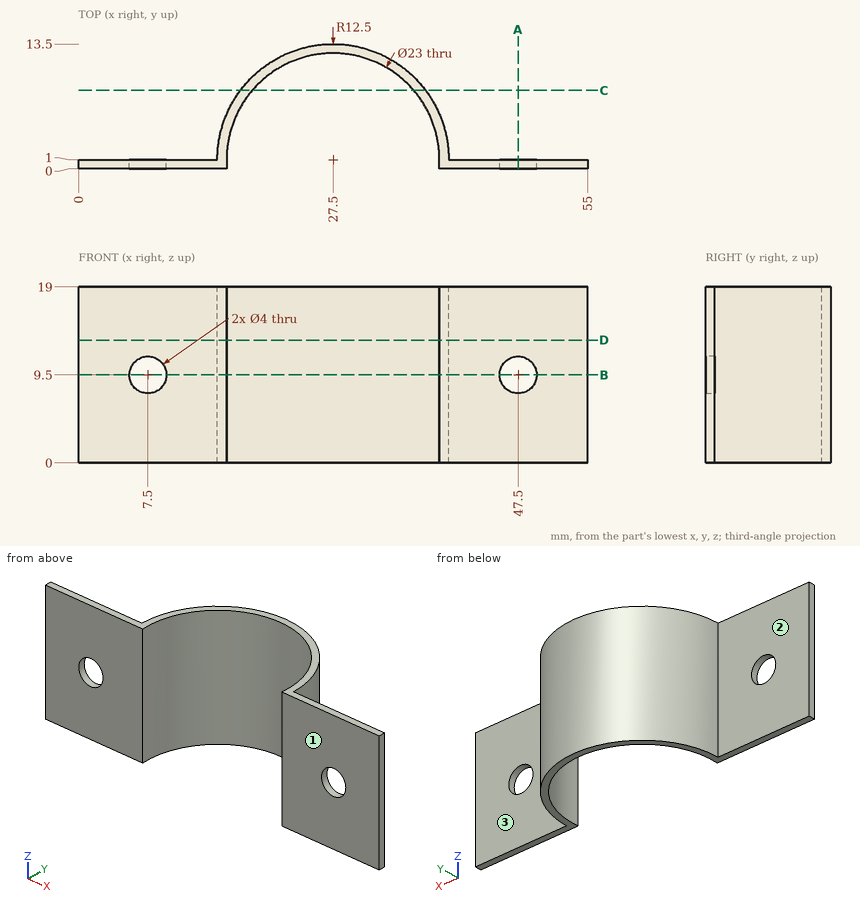
Job drawing, mm, ordinate dimensions from the low corner. One solid piece. A direction names the side the tool comes from. Give positions to 0.01 mm unless a question says otherwise; leave off trailing zeros. Write each loop counter-clockwise with the first axis right and the second up, starting at its lowest first coordinate (ties: lowest second). Pieces come first, ordered by that corner, then holes. Notation, with made-up numbers: M -21,-38.75 L 8,-38.75 A30 ccw 8,-4.75 Z; hole C 65,38.25 d7. An arc over 180 degrees is marked long. Put each result on its own line as item: value. Start each with the question number.
(1) Band-saw the part on B-B, the plane z = 9.5. Write the cut outline in (x, y), and give its area (3 significant figures).
(2) Band-saw the part on D-D, the plane z = 13.25. Write the cut outline in (x, y).
(3) Probe L1, parallel to X at y = 0.65, z = 9.5; L2, parallel to Y at x = 8, z = 4; L3, parallel to X at y = 4.75, z = 5.25. List the from-to ranges inside material, lowest first.
(4) Which spindle directions (+Z, -Z, +X, -X, +Y, -Y) get a long thin tool onto all of the face, cutting with end or side? Do the marked faces 1, 2 and 3. Say none if no direction does.
(5) Flat gauge pins, fed straight in: pin 1 Ø1.5 at (y, z) = (3, 15) entering from -X; pin 2 Ø2 at (y, z) = (9, 7.5) entering from -X; pin 3 Ø4 at (x, z) = (46, 9.5) entering from +Y. Where does each tip first touch, or does it go through?
(6) Band-saw the part on A-A, the plane x = 47.5. Write the cut outline in (y, z).
(7) Band-saw the part on C-C, the plane y = 8.5. Write the cut outline in (x, z), and give its area (3 significant figures).
Response values:
1. outline: M 0,0 L 5.5,0 L 5.5,1 L 0,1 Z; M 9.5,0 L 16.04,0 A11.5 cw long 38.96,0 L 45.5,0 L 45.5,1 L 40,1 A12.5 ccw 15,1 L 9.5,1 Z; M 49.5,0 L 55,0 L 55,1 L 49.5,1 Z
1. area: 61.7 mm2
2. outline: M 0,0 L 16.04,0 A11.5 cw long 38.96,0 L 55,0 L 55,1 L 40,1 A12.5 ccw 15,1 L 0,1 Z
3. L1: x = 0 to 5.5, 9.5 to 16.01, 38.99 to 45.5, 49.5 to 55
3. L2: y = 0 to 1
3. L3: x = 15.58 to 16.63, 38.37 to 39.42
4. face 1: +Z, -Z, +X, -X, -Y
4. face 2: +Z, -Z, -X, +Y
4. face 3: +Z, -Z, +X, +Y
5. pin 1: stops at x = 15.06
5. pin 2: stops at x = 17.14
5. pin 3: stops at y = 1
6. outline: M 0,0 L 1,0 L 1,7.5 L 0,7.5 Z; M 0,11.5 L 1,11.5 L 1,19 L 0,19 Z
7. outline: M 17.5,0 L 18.78,0 L 18.78,19 L 17.5,19 Z; M 36.22,0 L 37.5,0 L 37.5,19 L 36.22,19 Z
7. area: 48.7 mm2
